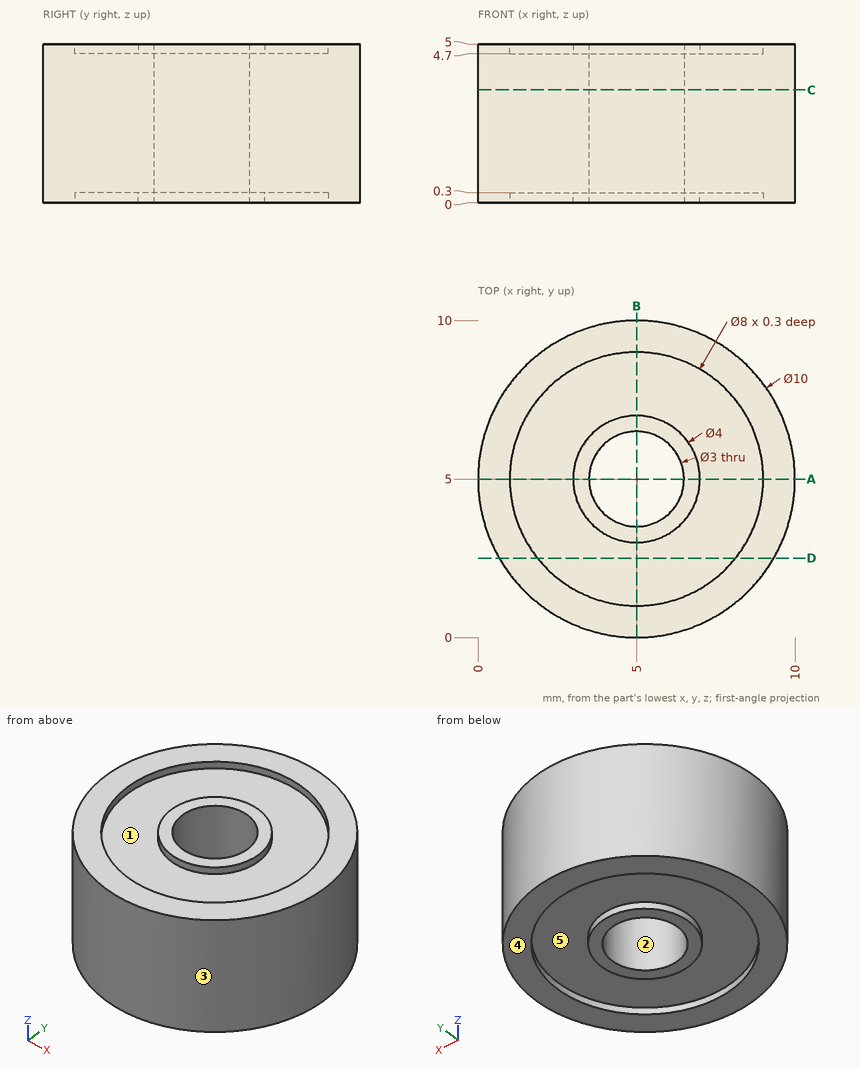
Geometry: see drawing. Coordinates: mm, zero at the bounding-box minimum. A direction names the side the tool comes from. Give positions to 0.01 mm unless a question says otherwise; leave off trailing zeros. Loops run counter-clockwise (first coordinate to the right, second up) from the corner with the lowest first, then second, coordinate; pieces in that order, holes last. Notation, with made-up numbers: (-4.75, -18) -> (32.25, -18) arc R21 ccw to (32.25, 18) -> close; hole circle Ø2 at (-6.75, -12). An arc over 180 degrees is marked (long way). Answer as a JSON object with one key per item and string values. Group by question number.
Item 1: Cut plane A-A, the plane y = 5. Return the cut outline in (x, z).
Item 2: Cut plane C-C, the plane z = 3.55. Return the cut outline in (x, y), and give its area (3 significant figures).
Item 3: Pin query (flat end, axial travel): P1, Ø2, axis at x = 9, z = 3, coming from the -Y side. Return the tip coordinate at first contact, or that it passes through.
Item 4: Line query: probe 1 along X at (y, z) = (5, 4.95); probe 2 along X at (y, z) = (5, 2.3). Output: solid intervals per line, ascending.
Item 5: Pull-direction query (Y, two-part tool) for the marked faces 3, 4 and 5; classes: released by +Y, released by -Y, zero draft, split by the parting line, or undercut.
Item 6: Cut plane D-D, the plane y = 2.5. Return the cut outline in (x, z), and give its area (3 significant figures).
Item 7: Reachability of the marked faces 1 and 2 from +Z, -Z, +X, -X, +Y, -Y: full face, straight path, thin tool, end or side. Return the list, or none.
Checks:
{
 "1": {"outline": "(0, 0) -> (1, 0) -> (1, 0.3) -> (3, 0.3) -> (3, 0) -> (3.5, 0) -> (3.5, 5) -> (3, 5) -> (3, 4.7) -> (1, 4.7) -> (1, 5) -> (0, 5) -> close; (6.5, 0) -> (7, 0) -> (7, 0.3) -> (9, 0.3) -> (9, 0) -> (10, 0) -> (10, 5) -> (9, 5) -> (9, 4.7) -> (7, 4.7) -> (7, 5) -> (6.5, 5) -> close"},
 "2": {"outline": "circle Ø10 at (5, 5); hole circle Ø3 at (5, 5)", "area": "71.5 mm²"},
 "3": {"P1": "stops at y = 1"},
 "4": {"probe 1": "x = 0 to 1, 3 to 3.5, 6.5 to 7, 9 to 10", "probe 2": "x = 0 to 3.5, 6.5 to 10"},
 "5": {"face 3": "split by the parting line", "face 4": "zero draft", "face 5": "undercut"},
 "6": {"outline": "(0.67, 0) -> (1.88, 0) -> (1.88, 0.3) -> (8.12, 0.3) -> (8.12, 0) -> (9.33, 0) -> (9.33, 5) -> (8.12, 5) -> (8.12, 4.7) -> (1.88, 4.7) -> (1.88, 5) -> (0.67, 5) -> close", "area": "39.6 mm²"},
 "7": {"face 1": "+Z", "face 2": "+Z, -Z"}
}
